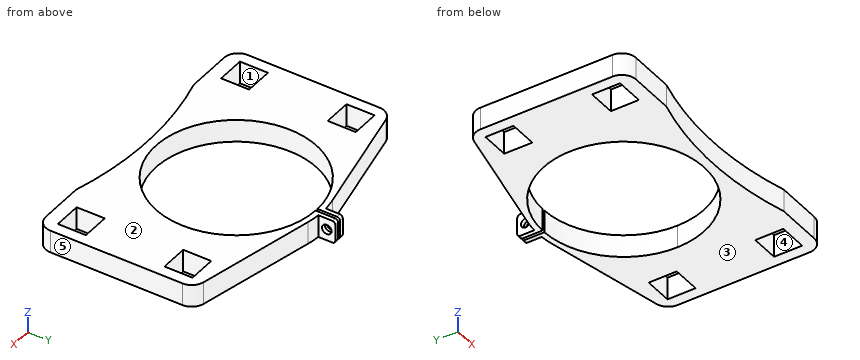
from build123d import *

# Parameters (mm, degrees)
SKIZZE1_R                       = 30.65
SKIZZE1_R_2                     = 28.65
AUFSATZ_LINEAR_AUSTRAGEN1_DEPTH = 8
AUFSATZ_LINEAR_AUSTRAGEN2_DEPTH = 8
SKIZZE3_W                       = 1
SKIZZE3_H                       = 2.855309686
SCHNITT_LINEAR_AUSTRAGEN1_DEPTH = 10
AUFSATZ_LINEAR_AUSTRAGEN3_DEPTH = 8
SKIZZE5_R                       = 1.7
SCHNITT_LINEAR_AUSTRAGEN2_DEPTH = 8
VERRUNDUNG2_R                   = 1
SKIZZE7_W                       = 10
SKIZZE7_H                       = 10
SCHNITT_LINEAR_AUSTRAGEN4_DEPTH = 10
VERRUNDUNG3_R                   = 5


with BuildPart() as part:
    # Skizze1 → Aufsatz-Linear austragen1 (new body)
    with BuildSketch(Plane.XY):
        Circle(SKIZZE1_R)
        Circle(SKIZZE1_R_2, mode=Mode.SUBTRACT)
    extrude(amount=AUFSATZ_LINEAR_AUSTRAGEN1_DEPTH)

    # Skizze2 → Aufsatz-Linear austragen2 (add)
    with BuildSketch(Plane.XY.offset(8)):
        with BuildLine():
            Line((52.5, -36.106090228), (52.5, 20))
            Line((52.5, 20), (6.481641536, 29.956815969))
            Line((6.481641536, 29.956815969), (6.460494255, 29.859077581))
            ThreePointArc((6.460494255, 29.859077581), (26.986544825, -14.318830203), (-21.103143411, -22.089812995))
            ThreePointArc((-21.103143411, -22.089812995), (-29.404257147, 8.288073457), (-6.460494255, 29.859077581))
            Line((-6.460494255, 29.859077581), (-6.481641536, 29.956815969))
            Line((-6.481641536, 29.956815969), (-52.5, 20))
            Line((-52.5, 20), (-52.5, -36.106090228))
            Line((-52.5, -36.106090228), (-31.288777705, -36.106090228))
            ThreePointArc((-31.288777705, -36.106090228), (0, -31.845839174), (31.288777705, -36.106090228))
            Line((31.288777705, -36.106090228), (52.5, -36.106090228))
        make_face()
    extrude(amount=-AUFSATZ_LINEAR_AUSTRAGEN2_DEPTH)

    # Skizze3 → Schnitt-Linear austragen1 (cut)
    with BuildSketch(Plane.XY.offset(8)):
        with Locations((0, 29.34103969)):
            Rectangle(SKIZZE3_W, SKIZZE3_H)
    extrude(amount=-SCHNITT_LINEAR_AUSTRAGEN1_DEPTH, mode=Mode.SUBTRACT)

    # Skizze4 → Aufsatz-Linear austragen3 (add)
    with BuildSketch(Plane.XY.offset(8)):
        Polygon((0.5, 30.645921425), (0.5, 36.645921425), (2, 36.645921425), (2, 29.02715443), align=None)
        Polygon((-2, 29.02715443), (-0.5, 30.645921425), (-0.5, 36.645921425), (-2, 36.645921425), align=None)
    extrude(amount=-AUFSATZ_LINEAR_AUSTRAGEN3_DEPTH)

    # Skizze5 → Schnitt-Linear austragen2 (cut)
    with BuildSketch(Plane.ZY.offset(2)):
        with Locations(Location((4, 33.615299481, 0), (0, 0, 270))):
            Circle(SKIZZE5_R)
    extrude(amount=-SCHNITT_LINEAR_AUSTRAGEN2_DEPTH, mode=Mode.SUBTRACT)

    # Verrundung2
    verrundung2_edges = [part.edges().sort_by_distance(p)[0] for p in [
        (1.25, 36.645921425, 8),
        (1.25, 36.645921425, 0),
        (-1.25, 36.645921425, 8),
        (-1.25, 36.645921425, 0),
    ]]
    fillet(verrundung2_edges, radius=VERRUNDUNG2_R)

    # Skizze7 → Schnitt-Linear austragen4 (cut)
    with BuildSketch(Plane(origin=(0, 0, 0), x_dir=(-1, 0, 0), z_dir=(0, 0, -1))):
        with Locations((-43.5, 11.86546468)):
            Rectangle(SKIZZE7_W, SKIZZE7_H)
        with Locations((-43.5, -26.13453532)):
            Rectangle(SKIZZE7_W, SKIZZE7_H)
        with Locations((43.5, -26.13453532)):
            Rectangle(SKIZZE7_W, SKIZZE7_H)
        with Locations((43.5, 11.86546468)):
            Rectangle(SKIZZE7_W, SKIZZE7_H)
    extrude(amount=-SCHNITT_LINEAR_AUSTRAGEN4_DEPTH, mode=Mode.SUBTRACT)

    # Verrundung3
    verrundung3_edges = [part.edges().sort_by_distance(p)[0] for p in [
        (52.5, 20, 4),
        (52.5, -36.106090228, 4),
        (-52.5, -36.106090228, 4),
        (-52.5, 20, 4),
    ]]
    fillet(verrundung3_edges, radius=VERRUNDUNG3_R)


solid = part.part
Geometry: final body of the model. Coordinates: model frame, mm. Face numbers are marked on the shaded views. A direction names the side the tool comes from. Round coordinates to 2 decimals unless told otherwise and drop trailing zeros. Write each loop counter-clockwise with the first axis right and the second up, starting at its lowest first coordinate (ties: lowest second). Pieces come first, ordered by that corner, then holes. Notation, with made-up numbers: M 38,88.5 L 61,88.5 A25 ccw 61,112.5 Z; hole C 78,5 d4. An arc over 180 degrees is marked long. Write item = value, one per line.
Item 1: Pin query (flat end, axial travel): P1, Ø4, axis at y = 33.62, z = 4, coming from the -X side; P2, Ø1, axis at x = -29, z = 3.5, coming from the -Y side (3 decimals). Return the tip coordinate at first contact, or that it passes through.
Findings:
P1 = -2
P2 = -35.625
Item 2: Material intervals for line 1 along X through (y, z) = (-30, 6); line 2 along X through (y, z) = (0, 2); line 3 along X through (y, z) = (10, 3), sorted ascending. Write a range as [from, to].
Findings:
line_1 = [-52.5, -48.5], [-38.5, 38.5], [48.5, 52.5]
line_2 = [-52.5, -28.65], [28.65, 52.5]
line_3 = [-52.5, -48.5], [-38.5, -26.85], [26.85, 38.5], [48.5, 52.5]
Item 3: Section query B-B on x = -8.5. Return loops of the section in (y, z).
Findings:
outline = M -32.15,0 L -27.36,0 L -27.36,8 L -32.15,8 Z; M 27.36,0 L 29.52,0 L 29.52,8 L 27.36,8 Z
Item 4: Access query for the marked faces 1 and 2. Directions: +Z, -Z, +X, -X, +Y, -Y. A direction counts if a zero-diameter tool reaches every point of the face in a straight line with its end or side. Return the directions, or none.
Findings:
face_1 = +Z, -Z
face_2 = +Z, +X, -X, +Y, -Y
Item 5: Section query A-A on y = -13.5. Return loops of the section in (x, z).
Findings:
outline = M -52.5,0 L -25.27,0 L -25.27,8 L -52.5,8 Z; M 25.27,0 L 52.5,0 L 52.5,8 L 25.27,8 Z
Item 6: Section query C-C on z = 4. State how many separate pieces and enclosed holes the cut face has, then the cut area to 3 significant figures.
Findings:
separate_pieces = 3
enclosed_holes = 4
area = 3,320 mm^2
Item 7: Pull-direction query (X, two-part tool) for the marked faces 3, 4 and 5; classes: pulls with the +X half, pulls with the -X half, needs draft (parallel to the pull), parting line crosses it, or undercut.
Findings:
face_3 = needs draft
face_4 = undercut
face_5 = pulls with the +X half
